The model under review builds one solid part; all positions refer to its coordinate system, in mm. A direction names the side the tool comes from. Coordinates: 2 decimals unless noted, no trailing zeros. Write each loop counter-clockwise with the first axis right and the second up, starting at its lowest first coordinate (ties: lowest second). Pieces come first, ordered by that corner, then holes.
1) Machinability: for faces 4 (the flat face through (0, -17, 33)), 5 (the flat face through (7.226, -22.185, 3.938)), 6 (the cylindrical face through (18, -9, 27)), which of the approach directions +Z, -Z, +X, -X, +Y, -Y give a long, thin tool a straight path to every point of the face, cutting with its end or side? Answer none if there is none.
2) Add section B-B, the plane y = -17.5. State the section outline as (x, z) points.
3) For P1, Ø4, axis at x = -13.5, z = 16.5, coming from the +Y side; P2, Ø2.5, axis at x = 0, y = -22.5, coming from the +Z side; P3, Ø13, axis at x = 0, z = 14, coming from the +Y side; P4, Ø5, axis at x = 6.5, y = -27, coming from the -Z side, all flat-tipped, find the tip position at first contact; note any pin that passes through.
4) Add section C-C, the plane z = 9. State the section outline as (x, y) points (3 decimals).
5) For line 1 (X direction, y = -37.5, z = 24.25); line 2 (Y direction, x = -16, z = 23); line 3 (Y direction, x = -18, z = 28.5), list the stretches that pass through material, from the lowest coordinate up.
6) Add section A-A, the plane x = 6. State the section outline as (y, z) points.
7) Mouldability with a two-part tool opening along Y and no side actions: class faces 1 (the conical face through (15.566, -7.481, 19.759)), 2 (the flat face through (-7.29, -22.18, 3.83)), 3 (the flat face through (-5.3, 0, 20.4)) as released by +Y, released by -Y, zero draft, split by the parting line, or undercut.
from build123d import *

# Parameters (mm, degrees)
F1_DEPTH       = 45
F5_D           = 5
F5_DEPTH       = 12
F5_CSINK_D     = 6
F5_CSINK_ANGLE = 80
F5_TIP         = 1.5021515476
F6_D           = 3
F6_DEPTH       = 5
F6_CSINK_D     = 3.5
F6_CSINK_ANGLE = 80
F6_TIP         = 0.9012909285


with BuildPart() as f1:
    # F0 (on Front) → F1 (new body)
    with BuildSketch(Plane.XZ):
        with BuildLine():
            Line((9.5, 0), (22.5, 0))
            Line((22.5, 0), (22.5, 33))
            Line((22.5, 33), (0, 33))
            Line((0, 33), (-22.5, 33))
            Line((-22.5, 33), (-22.5, 0))
            Line((-22.5, 0), (-9.5, 0))
            Line((-9.5, 0), (-5.0154756716, 7.7674239846))
            ThreePointArc((-5.0154756716, 7.7674239846), (-3.4551551794, 21.2153934533), (8, 14))
            ThreePointArc((8, 14), (7.2153934533, 10.5448448206), (5.0154756716, 7.7674239846))
            Line((5.0154756716, 7.7674239846), (9.5, 0))
        make_face()
    extrude(amount=F1_DEPTH)

    # F5
    with Locations(Plane.XY.offset(33)):
        with Locations((-16, -7.5), (-16, -37.5), (16, -37.5), (16, -7.5)):
            CounterSinkHole(F5_D / 2, F5_CSINK_D / 2, depth=F5_DEPTH, counter_sink_angle=F5_CSINK_ANGLE)
            with Locations((0, 0, -(F5_DEPTH + F5_TIP / 2))):  # 118° drill point
                Cone(0, F5_D / 2, F5_TIP, mode=Mode.SUBTRACT)

    # F6
    with Locations(Plane.XY.offset(33)):
        with Locations((0, -22.5)):
            CounterSinkHole(F6_D / 2, F6_CSINK_D / 2, depth=F6_DEPTH, counter_sink_angle=F6_CSINK_ANGLE)
            with Locations((0, 0, -(F6_DEPTH + F6_TIP / 2))):  # 118° drill point
                Cone(0, F6_D / 2, F6_TIP, mode=Mode.SUBTRACT)


solid = f1.part
Geometry results:
1. face 4: +Z, +X, -X, +Y, -Y
1. face 5: -Z, +Y, -Y
1. face 6: +Z
2. outline: (-22.5, 0) - (-9.5, 0) - (-5.02, 7.77) arc R8 cw (long way) to (5.02, 7.77) - (9.5, 0) - (22.5, 0) - (22.5, 33) - (-22.5, 33) - close
3. P1: stops at y = 0
3. P2: stops at z = 27.85
3. P3: passes through
3. P4: stops at z = 0.87
4. outline: (-22.5, -45) - (-6.245, -45) - (-6.245, 0) - (-22.5, 0) - close; (6.245, -45) - (22.5, -45) - (22.5, 0) - (6.245, 0) - close
5. line 1: x = -22.5 to -18.5, -13.5 to 13.5, 18.5 to 22.5
5. line 2: y = -45 to -40, -35 to -10, -5 to 0
5. line 3: y = -45 to -39, -36 to -9, -6 to 0
6. outline: (-45, 6.06) - (0, 6.06) - (0, 8.71) - (-45, 8.71) - close; (-45, 19.29) - (0, 19.29) - (0, 33) - (-45, 33) - close
7. face 1: undercut
7. face 2: zero draft
7. face 3: released by +Y
